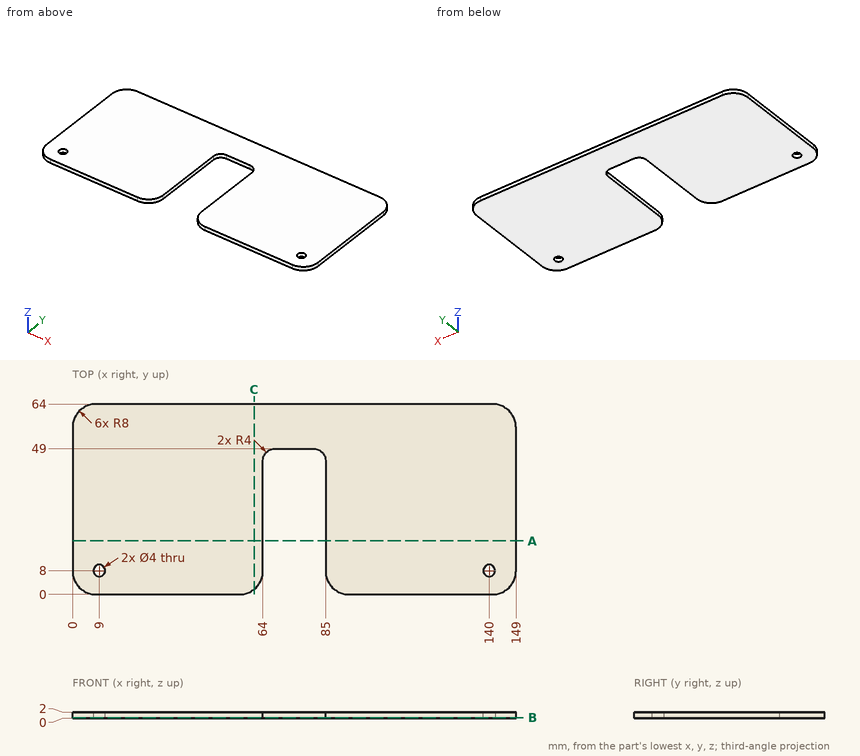
Part print with two shaded views. Sizes in mm from the minimum x, y, z corner. Coordinates: 2 decimals unless noted, no trailing zeros. Order: outer loops, then holes, each group sorted by start corner. A loop starts at its lowest first (then second) coordinate and runs counter-clockwise, first axis right, second up. Notation, with made-up numbers: M 40,44 L 83,44 A25 ccw 83,56 Z; hole C 62.5,-29 d8. An arc over 180 degrees is marked long. One line per question, with ' | ' between items. Start each with the question number.
1. Cut at C-C (x = 61). Write the cut outline in (y, z) (3 decimals), plus the area to 3 significant figures.
2. Wall check: line 1 along Y through (x, z) = (140, 0.85); line 2 along X through (y, z) = (21, 0.4); line 3 along X through (y, z) = (61.5, 1.7). Give the ranges that are in metal, low to high. Write a range as [from, to].
3. Cut at B-B (z = 0.3). Write the cut outline in (x, y), plus the area to 3 significant figures.
4. Flat gauge pins, fed straight in: P1, Ø3, axis at x = 140, y = 8, coming from the -Z side; P2, Ø1, axis at x = 76, z = 1, coming from the -Y side. Where does each tip first touch, or does it go through?
5. Cut at A-A (y = 18). Write the cut outline in (x, z), plus the area to 3 significant figures.
The answers:
1) outline: M 1.755,0 L 64,0 L 64,2 L 1.755,2 Z | area: 124 mm2
2) line 1: y = [0, 6], [10, 64] | line 2: x = [0, 64], [85, 149] | line 3: x = [2.19, 146.81]
3) outline: M 0,8 A8 ccw 8,0 L 56,0 A8 ccw 64,8 L 64,45 A4 cw 68,49 L 81,49 A4 cw 85,45 L 85,8 A8 ccw 93,0 L 141,0 A8 ccw 149,8 L 149,56 A8 ccw 141,64 L 8,64 A8 ccw 0,56 Z; hole C 9,8 d4; hole C 140,8 d4 | area: 8,410 mm2
4) P1: passes through | P2: stops at y = 49
5) outline: M 0,0 L 64,0 L 64,2 L 0,2 Z; M 85,0 L 149,0 L 149,2 L 85,2 Z | area: 256 mm2
